from build123d import *

# Parameters (mm, degrees)
BOSS_EXTRUDE1_DEPTH = 0.7874
SKETCH4_W           = 3.17
SKETCH4_H           = 4.61
BOSS_EXTRUDE3_DEPTH = 0.6
SKETCH2_W           = 1
SKETCH2_H           = 1
BOSS_EXTRUDE2_DEPTH = 0.1
SKETCH5_R           = 0.5
CUT_EXTRUDE1_DEPTH  = 1.7874


with BuildPart() as part:
    # Sketch1 → Boss-Extrude1 (new body)
    with BuildSketch(Plane(origin=(0, 0, 0), x_dir=(1, 0, 0), z_dir=(0, 1, 0))):
        Polygon((2, 3), (2, 1), (3, 1), (3, -4.5), (-2, -4.5), (-2, 3), align=None)
    extrude(amount=BOSS_EXTRUDE1_DEPTH)

    # Sketch4 → Boss-Extrude3 (add)
    with BuildSketch(Plane(origin=(0, 0.7874, 0), x_dir=(1, 0, 0), z_dir=(0, 1, 0))):
        with Locations((0, -0.635)):
            Rectangle(SKETCH4_W, SKETCH4_H)
    extrude(amount=BOSS_EXTRUDE3_DEPTH)

    # Sketch2 → Boss-Extrude2 (add)
    with BuildSketch(Plane(origin=(0, 1.3874, 0), x_dir=(1, 0, 0), z_dir=(0, 1, 0))):
        Rectangle(SKETCH2_W, SKETCH2_H)
    extrude(amount=BOSS_EXTRUDE2_DEPTH)

    # Sketch5 → Cut-Extrude1 (cut, through all)
    with BuildSketch(Plane(origin=(0, 0.7874, 0), x_dir=(1, 0, 0), z_dir=(0, 1, 0))):
        with Locations((2, -3.5)):
            Circle(SKETCH5_R)
    extrude(amount=-CUT_EXTRUDE1_DEPTH, mode=Mode.SUBTRACT)


solid = part.part
Input: part model. Units: mm. Frame: model coordinates. Coordinates: 2 decimals unless noted, no trailing zeros. Loops run counter-clockwise (first coordinate to the right, second up) from the corner with the lowest first, then second, coordinate; pieces in that order, holes last. Notation, with made-up numbers: (1.25, 20) -> (36.25, 20) arc R31 cw to (36.25, 50) -> close; hole circle Ø10 at (74.5, -9). An arc over 180 degrees is marked (long way). One line per item, written item: value.
(1) Cut plane A-A (z = 3.5). Output: boundary loops of the cut face in (x, y), then the cut area to 3 significant figures.
Answer below:
outline: (-2, 0) -> (1.5, 0) -> (1.5, 0.79) -> (-2, 0.79) -> close; (2.5, 0) -> (3, 0) -> (3, 0.79) -> (2.5, 0.79) -> close
area: 3.15 mm2
(2) Pin query (flat end, axial travel): pin 1 Ø0.6 at (y, z) = (0.5, -1.5) entering from +X; pin 2 Ø2.5 at (x, z) = (0, 2) entering from +Y. Return the tip coordinate at first contact, or that it passes through.
Answer below:
pin 1: stops at x = 2
pin 2: stops at y = 1.39
(3) Ray query, line 1 along X through (y, z) = (0.2, 3.5); line 2 along Y through (x, z) = (0.9, 0.25); line 3 along Y through (x, z) = (2.55, 2.75). Return the intervals inside material, ascending.
Answer below:
line 1: x = -2 to 1.5, 2.5 to 3
line 2: y = 0 to 1.39
line 3: y = 0 to 0.79
(4) Draft query along X for faces 1 (the face through (1.6, 0.4, 3.2)), 2 (the face through (0, 1.387, 1)). Return one class per face: pulls with the +X half, pulls with the -X half, needs draft (parallel to the pull), parting line crosses it, or undercut.
Answer below:
face 1: undercut
face 2: needs draft
(5) Cut plane D-D (x = -1.3). Output: boundary loops of the cut face in (y, z), then the cut area to 3 significant figures.
Answer below:
outline: (0, -3) -> (0.79, -3) -> (0.79, -1.67) -> (1.39, -1.67) -> (1.39, 2.94) -> (0.79, 2.94) -> (0.79, 4.5) -> (0, 4.5) -> close
area: 8.67 mm2
(6) Cut plane C-C (x = 1.9). Output: boundary loops of the cut face in (y, z).
Answer below:
outline: (0, -3) -> (0.79, -3) -> (0.79, 3.01) -> (0, 3.01) -> close; (0, 3.99) -> (0.79, 3.99) -> (0.79, 4.5) -> (0, 4.5) -> close
(7) Cut plane B-B (y = 0.35). Output: boundary loops of the cut face in (x, z).
Answer below:
outline: (-2, -3) -> (2, -3) -> (2, -1) -> (3, -1) -> (3, 4.5) -> (-2, 4.5) -> close; hole circle Ø1 at (2, 3.5)
